Check sheet for the modelled part. Datum: model origin and axes. Units: mm. A direction names the side the tool comes from. Coordinates: 2 decimals unless noted, no trailing zeros. Loops run counter-clockwise (first coordinate to the right, second up) from the corner with the lowest first, then second, coordinate; pieces in that order, holes last. Notation, with made-up numbers: M 80,37.25 L 138,37.25 A30 cw 138,61.25 Z; hole C 55,64.25 d7. An arc over 180 degrees is marked long. Return JSON: item names as keys, results as strings.
Autodesk Inventor part; units mm, degrees
ref_plane "YZ Plane" through (0, 0, 0) normal (1, 0, 0) x (0, 1, 0)
ref_plane "XZ Plane" through (0, 0, 0) normal (0, 1, 0) x (-1, 0, 0)
ref_plane "XY Plane" through (0, 0, 0) normal (0, 0, 1) x (1, 0, 0)
sketch "Sketch1" plane through (0, 0, 0) normal (1, 0, 0) x (0, 1, 0)
  line L0 (0, 0) -> (50.8, 0)
  line L1 (50.8, 0) -> (50.8, -25.4)
  line L2 (50.8, -25.4) -> (0, -25.4)
  line L3 (0, -25.4) -> (0, 0)
  line L4 (3.175, -3.175) -> (47.625, -3.175)
  line L5 (47.625, -3.175) -> (47.625, -22.225)
  line L6 (47.625, -22.225) -> (3.175, -22.225)
  line L7 (3.175, -22.225) -> (3.175, -3.175)
  dimension "d0" = 50.8
  dimension "d1" = 25.4
  dimension "d2" = 44.45
  dimension "d3" = 19.05
  dimension "d4" = 3.175
  dimension "d5" = 3.175
extrude "Extrusion1" add sketch "Sketch1" along normal blind 63.5
sketch "Sketch2" plane through (0, 50.8, 0) normal (0, 1, 0) x (1, 0, 0)
  line L0 (0, 0) -> (63.5, 0)
  line L1 (63.5, 25.4) -> (63.5, 0)
  point P0 (57.15, 12.7)
  point P1 (31.75, 12.7)
  point P2 (6.35, 12.7)
  dimension "d8" = 6.35
  dimension "d9" = 31.75
  dimension "d10" = 57.15
  dimension "d11" = 12.7
  dimension "d12" = 12.7
  dimension "d13" = 12.7
hole "Hole1" at (57.15, 50.8, -12.7) at (31.75, 50.8, -12.7) at (6.35, 50.8, -12.7) direction (0, -1, 0) diameter 6.35 end through all
properties part number "back roller 2x1"
1) Section check C-C on z = -12.7. Count the separate pieces of the cut face and the enclosed holes in it, then the cut area to 3 significant figures.
Answers:
{"separate pieces": "8", "enclosed holes": "0", "area": "282 mm²"}
2) Section check D-D on x = 57.15. Record the cut outline in (y, z) (3 decimals).
Answers:
{"outline": "M 0,-25.4 L 50.8,-25.4 L 50.8,-15.875 L 47.625,-15.875 L 47.625,-22.225 L 3.175,-22.225 L 3.175,-15.875 L 0,-15.875 Z; M 0,-9.525 L 3.175,-9.525 L 3.175,-3.175 L 47.625,-3.175 L 47.625,-9.525 L 50.8,-9.525 L 50.8,0 L 0,0 Z"}
3) Section check A-A on y = 46. Record the cut outline in (x, z) (3 decimals).
Answers:
{"outline": "M 0,-25.4 L 63.5,-25.4 L 63.5,-22.225 L 0,-22.225 Z; M 0,-3.175 L 63.5,-3.175 L 63.5,0 L 0,0 Z"}
4) Draft check along X on faces 3 (the face through (0, 25, -2)), 4 (the face through (31, 3.175, -17)), 5 (the face through (34.85, 49.19, -13.39)). Enter one of: +X half, -X half, draft (parallel to the pull), parting line (faces both ways), or undercut.
Answers:
{"face 3": "-X half", "face 4": "draft", "face 5": "undercut"}
5) Scan lines: line 1 along X through (y, z) = (0.9, -12.7) (3 decimals); line 2 along Z through (x, y) = (48, 43.5) (3 decimals); line 3 along Z through (x, y) = (6.35, 49) (3 decimals). Record each from-to range of solid material in increasing order. Write a range as [from, to].
Answers:
{"line 1": "[0, 3.175], [9.525, 28.575], [34.925, 53.975], [60.325, 63.5]", "line 2": "[-25.4, -22.225], [-3.175, 0]", "line 3": "[-25.4, -15.875], [-9.525, 0]"}
6) Set-up check for faces 1 (the face through (9.45, 1.57, -13.39)), 2 (the face through (31, 47.625, -8)): record each of +Z, -Z, +X, -X, +Y, -Y from which the full face is reachable in a straight line by a thin tool's end or side.
Answers:
{"face 1": "+Y, -Y", "face 2": "+X, -X"}
7) Section check B-B on z = -8.5. Record the cut outline in (x, y) (3 decimals), then the cut area to 3 significant figures.
Answers:
{"outline": "M 0,0 L 63.5,0 L 63.5,3.175 L 0,3.175 Z; M 0,47.625 L 63.5,47.625 L 63.5,50.8 L 0,50.8 Z", "area": "403 mm²"}
